Build history of the part. All positions in model axes, mm. A direction names the side the tool comes from. Give positions to 0.01 mm unless a question says otherwise; leave off trailing zeros. Loops run counter-clockwise (first coordinate to the right, second up) from the corner with the lowest first, then second, coordinate; pieces in that order, holes last. Notation, with made-up numbers: (55, 73) - (65, 73) arc R17 cw to (65, 79) - close; hole circle Ø3 at (48.25, 65.25). An arc over 180 degrees is marked (long way). Return JSON: item names as keys, results as strings. Group by question number.
1) Mould opens along Z. For faces 4 (the face through (-0.2, -2.3, 25.4)), 5 (the face through (4.999, 10, 13)), 6 (the face through (10.937, 0.542, 12.558)), 7 (the face through (7.33, 3.93, 24.11)) say: released by +Z, released by -Z, zero draft, split by the parting line, or undercut.
2) Slice it at B-B (y = 5.5). Count the separate pieces of the cut face and the enclosed holes in it, and give its area (3 significant figures).
3) 3-axis set-ups, long thin cutter, end or side, ignore diameter. For faces 1 (the face through (2.49, -1.62, 24.11)), 2 (the face through (5.94, 9.2, 12.84)), 3 (the face through (-3.994, -9, 13)): which of +Z, -Z, +X, -X, +Y, -Y reach the whole face in a straight line?
4) Drill centre lines: probe 1 along Z at (x, y) = (7.5, -5); probe 2 along Y at (x, z) = (-5, 5.75); probe 3 along Y at (x, z) = (5.5, 10.5). Where is each one in solid material? Low to high. Write a range as from..to.
5) Slice it at A-A (z = 13). List the corners of the cut face in (x, y).
6) Slice it at D-D (y = 9). List the corners of the cut face in (x, z).
7) Slice it at C-C (x = -8.25). List the corners of the cut face in (y, z).
8) Drop flat-ended pins along their axis: pin 1 (8 mm diameter, centred on y = -0.5, z = 4.5, fed in from -X); pin 2 (1.5 mm diameter, centred on y = 7.5, z = 19, fed in from -X); pin 3 (1.4 mm diameter, centred on y = -9.5, z = 13.5, fed in from +X). Give the stop position or say it passes through.
```python
from build123d import *

# Parameters (mm, degrees)
F2_DEPTH = 25.4
F3_W     = 8.992830546
F3_H     = 20.32
F4_DEPTH = 21.7172655679
F6_DEPTH = 27.1463319599
F8_DEPTH = 27.1463319599


with BuildPart() as f2:
    # F1 (on face) → F2 (new body)
    with BuildSketch(Plane.XY):
        Polygon((12.5378917714, 0), (6.2689458857, 10.858132784), (-6.2689458857, 10.858132784), (-12.5378917714, 0), (-6.2689458857, -10.858132784), (6.2689458857, -10.858132784), align=None)
        Polygon((-3.0813198537, -0.8107819997), (-1.428119345, -3.1018054447), (-5.3015932459, -7.7946673792), (-8.9699157746, -0.8107819997), align=None, mode=Mode.SUBTRACT)
        Polygon((3.3147766868, -8.4572770768), (-3.2382511436, -8.1953331628), (0, -4.2720679194), align=None, mode=Mode.SUBTRACT)
        Polygon((-9.0911711595, 1.1845681444), (-4.9708869394, 7.7049685974), (-1.428119345, 3.4170282109), (-2.9231349472, 1.1845681444), align=None, mode=Mode.SUBTRACT)
        Polygon((0, 4.7049229033), (-3.0929306056, 8.4484092324), (3.0869638225, 8.2013805647), align=None, mode=Mode.SUBTRACT)
        Polygon((-1.4994712546, 0), (0, 2.0553264767), (1.5851336066, 0), (0, -1.9388410728), align=None, mode=Mode.SUBTRACT)
        Polygon((1.1896715732, 3.32692286), (5.1308790649, 8.1196792242), (9.5972880112, -0.3836320019), (4.8747631368, -7.8570856971), (1.1896715732, -3.2043200918), (3.8246668436, 0), align=None, mode=Mode.SUBTRACT)
    extrude(amount=F2_DEPTH)

    # F3 (on face) → F4 (cut, through all)
    with BuildSketch(Plane.XZ.offset(10.858132784)):
        with Locations((0.5025306127, 12.7)):
            Rectangle(F3_W, F3_H)
    extrude(amount=-F4_DEPTH, mode=Mode.SUBTRACT)

    # F5 (on face) → F6 (cut, through all)
    with BuildSketch(Plane(origin=(-9.4034188286, -5.429066392, 0), x_dir=(0.5, -0.8660254038, 0), z_dir=(-0.8660254038, -0.5, 0))):
        Polygon((-4.9989458857, 22.86), (-4.9989458857, 2.54), (4.9989458857, 2.54), (4.9989458857, 22.86), (0, 22.86), align=None)
    extrude(amount=-F6_DEPTH, mode=Mode.SUBTRACT)

    # F7 (on face) → F8 (cut, through all)
    with BuildSketch(Plane(origin=(-9.4034188286, 5.429066392, 0), x_dir=(-0.5, -0.8660254038, 0), z_dir=(-0.8660254038, 0.5, 0))):
        Polygon((-4.9989458857, 22.86), (-4.9989458857, 12.7), (-4.9989458857, 2.54), (4.9989458857, 2.54), (4.9989458857, 12.7), (4.9989458857, 22.86), (0, 22.86), align=None)
    extrude(amount=-F8_DEPTH, mode=Mode.SUBTRACT)


solid = f2.part
```
Results:
{
 "1": {"face 4": "released by +Z", "face 5": "undercut", "face 6": "undercut", "face 7": "zero draft"},
 "2": {"separate pieces": "8", "enclosed holes": "0", "area": "54.0 mm2"},
 "3": {"face 1": "+Z, -Z", "face 2": "+X", "face 3": "+Y, -Y"},
 "4": {"probe 1": "0..2.54, 22.86..25.4", "probe 2": "-10.86..-8.66, 8.66..10.86", "probe 3": "-10.86..-8.95, 8.95..10.86"},
 "5": {"outline": "(-12.54, 0) - (-11.9, -1.1) - (-10, 0) - (-11.9, 1.1) - close; (-6.9, -9.76) - (-6.27, -10.86) - (-3.99, -10.86) - (-3.99, -8.08) - close; (-6.9, 9.76) - (-3.99, 8.08) - (-3.99, 10.86) - (-6.27, 10.86) - close; (5, -10.86) - (6.27, -10.86) - (6.9, -9.76) - (5, -8.66) - close; (5, 8.66) - (6.9, 9.76) - (6.27, 10.86) - (5, 10.86) - close; (10, 0) - (11.9, -1.1) - (12.54, 0) - (11.9, 1.1) - close"},
 "6": {"outline": "(-7.34, 0) - (7.34, 0) - (7.34, 2.54) - (5.59, 2.54) - (5.59, 22.86) - (7.34, 22.86) - (7.34, 25.4) - (-7.34, 25.4) - (-7.34, 22.86) - (-5.59, 22.86) - (-5.59, 2.54) - (-7.34, 2.54) - close; hole (-3.99, 2.54) - (5, 2.54) - (5, 22.86) - (-3.99, 22.86) - close"},
 "7": {"outline": "(-7.43, 0) - (-2.18, 0) - (-2.18, 2.54) - (-7.43, 2.54) - close; (-7.43, 22.86) - (-2.18, 22.86) - (-2.18, 25.4) - (-7.43, 25.4) - close; (-0.81, 0) - (1.18, 0) - (1.18, 2.54) - (-0.81, 2.54) - close; (-0.81, 22.86) - (1.18, 22.86) - (1.18, 25.4) - (-0.81, 25.4) - close; (2.52, 0) - (7.43, 0) - (7.43, 2.54) - (2.52, 2.54) - close; (2.52, 22.86) - (7.43, 22.86) - (7.43, 25.4) - (2.52, 25.4) - close"},
 "8": {"pin 1": "x = -12.54", "pin 2": "x = -4.29", "pin 3": "x = 6.9"}
}
